Work out the finished part from the listing and answer in its coordinate system (mm). A direction names the side the tool comes from. Round coordinates to 2 decimals unless told otherwise and drop trailing zeros. Write each loop counter-clockwise with the first axis right and the second up, starting at its lowest first coordinate (ties: lowest second). Pieces come first, ordered by that corner, then holes.
1. Find section A-A (z = 0). Write down the section's boundary in (x, y).
2. A tool of negligible diameter and unlimited length cuts with its end or side. For faces 1 (the face through (11.549, -9.981, 19.606)), 2 (the face through (11.451, 4.576, 19.284)), 3 (the face through (11.45, 18.29, 7.63)), from which of +Z, -Z, +X, -X, +Y, -Y can it reach the whole face along a straight path? Write none if from no direction.
3. Flat-ended cylindrical pins translate along their axes: pin 1 Ø3 at (x, z) = (12, 4.5) entering from +Y; pin 2 Ø2 at (x, z) = (13.5, -13) entering from +Y; pin 3 Ø1.5 at (x, y) = (12, 5.5) entering from +Z. Find the tip coordinate at first contact, or state that the pin passes through.
4. Straight lines are drawn through the part: probe 1 along Y at (x, z) = (12.5, -15); probe 2 along Z at (x, y) = (10, -19); probe 3 along Y at (x, z) = (13.75, -3). For each, find the intervals that lie inside material, in ascending order.
5. Determine the mould class of faces 4 (the face through (11.45, 5.42, 16.64)), 5 (the face through (11.55, -3.43, 21.73)), 6 (the face through (11.5, 17.5, 0)), 7 (the face through (8, -9, 9)) for opening direction Y: pulls with the +Y half, pulls with the -Y half, needs draft (parallel to the pull), parting line crosses it, or undercut.
6. Find section C-C (z = -18.5). Write down the section's boundary in (x, y), and give its area (3 significant figures).
```python
from build123d import *

# Parameters (mm, degrees)
BASPROSKE_W        = 15
BASPROSKE_H        = 22
TOOTHCUT_DEPTH     = 35.539832078
TEETHCUTS_COUNT    = 20
TEETHCUTS_ANGLE    = 342
BORSKE_R           = 0.5
BORE_DEPTH         = 50.0000508
SKETCH1_R          = 11.1
CUT_EXTRUDE1_DEPTH = 16
CUT_EXTRUDE2_DEPTH = 8


with BuildPart() as part:
    # BasProSke → Base-Revolve (revolve)
    with BuildSketch(Plane(origin=(0, 0, 0), x_dir=(1, 0, 0), z_dir=(0, 1, 0)), mode=Mode.PRIVATE) as base_revolve_sk:
        with Locations((7.5, 11)):
            Rectangle(BASPROSKE_W, BASPROSKE_H)
    revolve(base_revolve_sk.sketch.rotate(Axis((-10, 0, 0), (1, 0, 0)), 180), axis=Axis((-10, 0, 0), (1, 0, 0)))

    # TooCutSke → ToothCut (cut, through all)
    with BuildSketch(Plane(origin=(0, 0, 0), x_dir=(0, 0, -1), z_dir=(1, 0, 0))):
        with BuildLine():
            ThreePointArc((0.986171591, 17.471189616), (0, 17.499), (-0.986171591, 17.471189616))
            ThreePointArc((-0.986171591, 17.471189616), (-1.626916196, 19.798789858), (-2.932850173, 21.829260982))
            ThreePointArc((-2.932850173, 21.829260982), (0, 22.0254), (2.932850173, 21.829260982))
            ThreePointArc((2.932850173, 21.829260982), (1.626916196, 19.798789858), (0.986171591, 17.471189616))
        make_face()
    toothcut = extrude(amount=TOOTHCUT_DEPTH, mode=Mode.SUBTRACT)

    # TeethCuts: ToothCut ×20 about axis
    teethcuts_axis = Axis((-10, 0, 0), (1, 0, 0))
    for i in range(1, TEETHCUTS_COUNT):
        add(toothcut.rotate(teethcuts_axis, i * TEETHCUTS_ANGLE / (TEETHCUTS_COUNT - 1)), mode=Mode.SUBTRACT)

    # BorSke → Bore (cut, symmetric)
    with BuildSketch(Plane(origin=(0, 0, 0), x_dir=(0, 0, -1), z_dir=(1, 0, 0))):
        with Locations(Location((0, 0, 0), (0, 0, 180))):
            Circle(BORSKE_R)
    extrude(amount=BORE_DEPTH, both=True, mode=Mode.SUBTRACT)

    # Sketch1 → Cut-Extrude1 (cut)
    with BuildSketch(Plane.ZY):
        Circle(SKETCH1_R)
    extrude(amount=-CUT_EXTRUDE1_DEPTH, mode=Mode.SUBTRACT)

    # Sketch2 → Cut-Extrude2 (cut)
    with BuildSketch(Plane.ZY):
        with BuildLine():
            ThreePointArc((17.471189616, 0.986171591), (19.784848102, 1.620704589), (21.806333941, 2.912696354))
            ThreePointArc((21.806333941, 2.912696354), (21.729143493, 3.441558231), (21.639128664, 3.968388926))
            ThreePointArc((21.639128664, 3.968388926), (19.317333972, 4.572472634), (16.920832513, 4.460989585))
            ThreePointArc((16.920832513, 4.460989585), (16.642537979, 5.407488385), (16.31134495, 6.336799421))
            ThreePointArc((16.31134495, 6.336799421), (18.31568345, 7.655235955), (19.838983319, 9.50866662))
            ThreePointArc((19.838983319, 9.50866662), (19.602143532, 9.987790994), (19.353734704, 10.461020648))
            ThreePointArc((19.353734704, 10.461020648), (16.958904602, 10.318064378), (14.714146429, 9.471478019))
            ThreePointArc((14.714146429, 9.471478019), (14.156988385, 10.28565413), (13.554832194, 11.067137173))
            ThreePointArc((13.554832194, 11.067137173), (15.05365209, 12.940419489), (15.929654782, 15.173862347))
            ThreePointArc((15.929654782, 15.173862347), (15.556349186, 15.556349186), (15.173862347, 15.929654782))
            ThreePointArc((15.173862347, 15.929654782), (12.940419489, 15.05365209), (11.067137173, 13.554832194))
            ThreePointArc((11.067137173, 13.554832194), (10.28565413, 14.156988385), (9.471478019, 14.714146429))
            ThreePointArc((9.471478019, 14.714146429), (10.318064378, 16.958904602), (10.461020648, 19.353734704))
            ThreePointArc((10.461020648, 19.353734704), (9.987790994, 19.602143532), (9.50866662, 19.838983319))
            ThreePointArc((9.50866662, 19.838983319), (7.655235955, 18.31568345), (6.336799421, 16.31134495))
            ThreePointArc((6.336799421, 16.31134495), (5.407488385, 16.642537979), (4.460989585, 16.920832513))
            ThreePointArc((4.460989585, 16.920832513), (4.572472634, 19.317333972), (3.968388926, 21.639128664))
            ThreePointArc((3.968388926, 21.639128664), (3.441558231, 21.729143493), (2.912696354, 21.806333941))
            ThreePointArc((2.912696354, 21.806333941), (1.620704589, 19.784848102), (0.986171591, 17.471189616))
            ThreePointArc((0.986171591, 17.471189616), (0, 17.499), (-0.986171591, 17.471189616))
            ThreePointArc((-0.986171591, 17.471189616), (-1.620704589, 19.784848102), (-2.912696354, 21.806333941))
            ThreePointArc((-2.912696354, 21.806333941), (-3.441558231, 21.729143493), (-3.968388926, 21.639128664))
            ThreePointArc((-3.968388926, 21.639128664), (-4.572472634, 19.317333972), (-4.460989585, 16.920832513))
            ThreePointArc((-4.460989585, 16.920832513), (-5.407488385, 16.642537979), (-6.336799421, 16.31134495))
            ThreePointArc((-6.336799421, 16.31134495), (-7.655235955, 18.31568345), (-9.50866662, 19.838983319))
            ThreePointArc((-9.50866662, 19.838983319), (-9.987790994, 19.602143532), (-10.461020648, 19.353734704))
            ThreePointArc((-10.461020648, 19.353734704), (-10.318064378, 16.958904602), (-9.471478019, 14.714146429))
            ThreePointArc((-9.471478019, 14.714146429), (-10.28565413, 14.156988385), (-11.067137173, 13.554832194))
            ThreePointArc((-11.067137173, 13.554832194), (-12.940419489, 15.05365209), (-15.173862347, 15.929654782))
            ThreePointArc((-15.173862347, 15.929654782), (-15.556349186, 15.556349186), (-15.929654782, 15.173862347))
            ThreePointArc((-15.929654782, 15.173862347), (-15.05365209, 12.940419489), (-13.554832194, 11.067137173))
            ThreePointArc((-13.554832194, 11.067137173), (-14.156988385, 10.28565413), (-14.714146429, 9.471478019))
            ThreePointArc((-14.714146429, 9.471478019), (-16.958904602, 10.318064378), (-19.353734704, 10.461020648))
            ThreePointArc((-19.353734704, 10.461020648), (-19.602143532, 9.987790994), (-19.838983319, 9.50866662))
            ThreePointArc((-19.838983319, 9.50866662), (-18.31568345, 7.655235955), (-16.31134495, 6.336799421))
            ThreePointArc((-16.31134495, 6.336799421), (-16.642537979, 5.407488385), (-16.920832513, 4.460989585))
            ThreePointArc((-16.920832513, 4.460989585), (-19.317333972, 4.572472634), (-21.639128664, 3.968388926))
            ThreePointArc((-21.639128664, 3.968388926), (-21.729143493, 3.441558231), (-21.806333941, 2.912696354))
            ThreePointArc((-21.806333941, 2.912696354), (-19.784848102, 1.620704589), (-17.471189616, 0.986171591))
            ThreePointArc((-17.471189616, 0.986171591), (-17.499, 0), (-17.471189616, -0.986171591))
            ThreePointArc((-17.471189616, -0.986171591), (-19.784848102, -1.620704589), (-21.806333941, -2.912696354))
            ThreePointArc((-21.806333941, -2.912696354), (-21.729143493, -3.441558231), (-21.639128664, -3.968388926))
            ThreePointArc((-21.639128664, -3.968388926), (-19.317333972, -4.572472634), (-16.920832513, -4.460989585))
            ThreePointArc((-16.920832513, -4.460989585), (-16.642537979, -5.407488385), (-16.31134495, -6.336799421))
            ThreePointArc((-16.31134495, -6.336799421), (-18.31568345, -7.655235955), (-19.838983319, -9.50866662))
            ThreePointArc((-19.838983319, -9.50866662), (-19.602143532, -9.987790994), (-19.353734704, -10.461020648))
            ThreePointArc((-19.353734704, -10.461020648), (-16.958904602, -10.318064378), (-14.714146429, -9.471478019))
            ThreePointArc((-14.714146429, -9.471478019), (-14.156988385, -10.28565413), (-13.554832194, -11.067137173))
            ThreePointArc((-13.554832194, -11.067137173), (-15.05365209, -12.940419489), (-15.929654782, -15.173862347))
            ThreePointArc((-15.929654782, -15.173862347), (-15.556349186, -15.556349186), (-15.173862347, -15.929654782))
            ThreePointArc((-15.173862347, -15.929654782), (-12.940419489, -15.05365209), (-11.067137173, -13.554832194))
            ThreePointArc((-11.067137173, -13.554832194), (-10.28565413, -14.156988385), (-9.471478019, -14.714146429))
            ThreePointArc((-9.471478019, -14.714146429), (-10.318064378, -16.958904602), (-10.461020648, -19.353734704))
            ThreePointArc((-10.461020648, -19.353734704), (-9.987790994, -19.602143532), (-9.50866662, -19.838983319))
            ThreePointArc((-9.50866662, -19.838983319), (-7.655235955, -18.31568345), (-6.336799421, -16.31134495))
            ThreePointArc((-6.336799421, -16.31134495), (-5.407488385, -16.642537979), (-4.460989585, -16.920832513))
            ThreePointArc((-4.460989585, -16.920832513), (-4.572472634, -19.317333972), (-3.968388926, -21.639128664))
            ThreePointArc((-3.968388926, -21.639128664), (-3.441558231, -21.729143493), (-2.912696354, -21.806333941))
            ThreePointArc((-2.912696354, -21.806333941), (-1.620704589, -19.784848102), (-0.986171591, -17.471189616))
            ThreePointArc((-0.986171591, -17.471189616), (0, -17.499), (0.986171591, -17.471189616))
            ThreePointArc((0.986171591, -17.471189616), (1.620704589, -19.784848102), (2.912696354, -21.806333941))
            ThreePointArc((2.912696354, -21.806333941), (3.441558231, -21.729143493), (3.968388926, -21.639128664))
            ThreePointArc((3.968388926, -21.639128664), (4.572472634, -19.317333972), (4.460989585, -16.920832513))
            ThreePointArc((4.460989585, -16.920832513), (5.407488385, -16.642537979), (6.336799421, -16.31134495))
            ThreePointArc((6.336799421, -16.31134495), (7.655235955, -18.31568345), (9.50866662, -19.838983319))
            ThreePointArc((9.50866662, -19.838983319), (9.987790994, -19.602143532), (10.461020648, -19.353734704))
            ThreePointArc((10.461020648, -19.353734704), (10.318064378, -16.958904602), (9.471478019, -14.714146429))
            ThreePointArc((9.471478019, -14.714146429), (10.28565413, -14.156988385), (11.067137173, -13.554832194))
            ThreePointArc((11.067137173, -13.554832194), (12.940419489, -15.05365209), (15.173862347, -15.929654782))
            ThreePointArc((15.173862347, -15.929654782), (15.556349186, -15.556349186), (15.929654782, -15.173862347))
            ThreePointArc((15.929654782, -15.173862347), (15.05365209, -12.940419489), (13.554832194, -11.067137173))
            ThreePointArc((13.554832194, -11.067137173), (14.156988385, -10.28565413), (14.714146429, -9.471478019))
            ThreePointArc((14.714146429, -9.471478019), (16.958904602, -10.318064378), (19.353734704, -10.461020648))
            ThreePointArc((19.353734704, -10.461020648), (19.602143532, -9.987790994), (19.838983319, -9.50866662))
            ThreePointArc((19.838983319, -9.50866662), (18.31568345, -7.655235955), (16.31134495, -6.336799421))
            ThreePointArc((16.31134495, -6.336799421), (16.642537979, -5.407488385), (16.920832513, -4.460989585))
            ThreePointArc((16.920832513, -4.460989585), (19.317333972, -4.572472634), (21.639128664, -3.968388926))
            ThreePointArc((21.639128664, -3.968388926), (21.729143493, -3.441558231), (21.806333941, -2.912696354))
            ThreePointArc((21.806333941, -2.912696354), (19.784848102, -1.620704589), (17.471189616, -0.986171591))
            ThreePointArc((17.471189616, -0.986171591), (17.499, 0), (17.471189616, 0.986171591))
        make_face()
    extrude(amount=-CUT_EXTRUDE2_DEPTH, mode=Mode.SUBTRACT)


solid = part.part
```
Worked answers:
1. outline: (8, -17.5) - (15, -17.5) - (15, -11.1) - (8, -11.1) - close; (8, 11.1) - (15, 11.1) - (15, 17.5) - (8, 17.5) - close
2. face 1: +Z, +X, -X, -Y
2. face 2: +X, -X
2. face 3: +X, -X, +Y
3. pin 1: stops at y = 21.79
3. pin 2: stops at y = 15.57
3. pin 3: stops at z = 16.84
4. probe 1: y = -15.89 to -12.85, -9.62 to 9.62, 12.85 to 15.89
4. probe 2: z = -10.49 to -8.35, -4.6 to -1.32, 1.32 to 4.6, 8.35 to 10.49
4. probe 3: y = -21.79 to -10.69, 10.69 to 21.79
5. face 4: undercut
5. face 5: pulls with the -Y half
5. face 6: pulls with the +Y half
5. face 7: needs draft
6. outline: (8, -10.49) - (15, -10.49) - (15, -7.83) - (8, -7.83) - close; (8, -4.62) - (15, -4.62) - (15, -1.18) - (8, -1.18) - close; (8, 1.18) - (15, 1.18) - (15, 4.62) - (8, 4.62) - close; (8, 7.83) - (15, 7.83) - (15, 10.49) - (8, 10.49) - close
6. area: 85.5 mm2
